Autodesk Inventor part; units mm, degrees
ref_plane "Work Plane1" through (33.5, 0, 0) normal (1, 0, 0) x (0, 1, 0)
ref_plane "XZ Plane" through (0, 0, 0) normal (0, 1, 0) x (-1, 0, 0)
ref_plane "XY Plane" through (0, 0, 0) normal (0, 0, 1) x (1, 0, 0)
sketch "Sketch1" plane through (0, 0, 0) normal (0, 1, 0) x (-1, 0, 0)
  circle A0 centre (0, 0) radius 33.5
  dimension "d0" = 67
extrude "Extrusion1" add sketch "Sketch1" along normal blind 6
ref_plane "Work Plane1" through (33.5, 0, 0) normal (1, 0, 0) x (0, 1, 0)
sketch "Sketch6" plane through (33.5, 0, 0) normal (1, 0, 0) x (0, 1, 0)
  line L0 (0, -33.5) -> (0, 33.5)
  point P0 (0, 0)
  point P1 (2.5, 0)
  dimension "d47" = 2.5
hole "Hole4" at (33.5, 2.5, 0) direction (-1, 0, 0) diameter 3 depth 8 tip angle 118
pattern_circular "Circular Pattern3" count 3 over 360 about axis through (0, 0, 0) along (0, 1, 0) of "Hole4"
sketch "Sketch7" plane through (0, 0, 0) normal (0, -1, 0) x (1, 0, 0)
  circle A0 centre (0, 0) radius 24.25
  circle A1 centre (0, 0) radius 33.5
  dimension "d58" = 48.5
  dimension "d59" = 67
extrude "Extrusion3" add sketch "Sketch7" along normal blind 3
chamfer "Chamfer1" distance 1.5 angle 45 1 edges at (-24.25, -3, 0)
sketch "Sketch8" plane through (0, 6, 0) normal (0, 1, 0) x (1, 0, 0)
  circle A0 centre (13.25, -22.9497) radius 1.5
  circle A1 centre (0, 0) radius 33.5 construction
  line L0 (0, 0) -> (13.25, -22.9497) construction
  line L1 (0, 0) -> (33.5, 0) construction
  dimension "d65" = 3
  dimension "d66" = 26.5
  dimension "d67" = 60
extrude "Extrusion4" cut sketch "Sketch8" against normal blind 10
pattern_circular "Circular Pattern4" count 3 over 360 about axis through (0, 0, 0) along (0, 1, 0) of "Extrusion4"
properties part number "Engine bulkhead" material "Steel AISI 1006 85 HR"
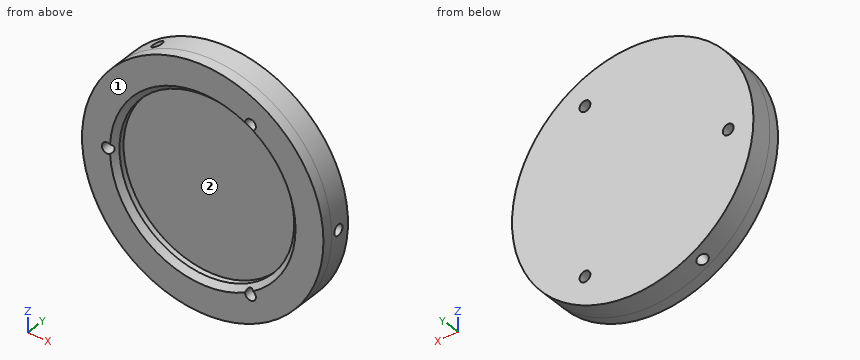
For this review, take the finished solid that the model builds, in its own axes (mm). Face numbers are marked on the shaded views. Round coordinates to 2 decimals unless told otherwise and drop trailing zeros. Loops run counter-clockwise (first coordinate to the right, second up) from the corner with the lowest first, then second, coordinate; pieces in that order, holes last. Notation, with made-up numbers: (-26.5, 55) - (4.5, 55) arc R31 ccw to (4.5, 79) - close; hole circle Ø1 at (88, 39.5). An arc over 180 degrees is marked (long way). Answer as CSV lines item,"result".
(1) Wall thickness on line 1 (Z direction, x = 13.25, y = 4.25); line 2 (X direction, y = 2.75, z = -23); line 3 (Z direction, x = 0, y = -1.1): over which ranges is each line inside the solid? List them lowest first.
Checked values:
line 1,"z = -30.77 to -24.45, -21.45 to 21.45, 24.45 to 30.77"
line 2,"x = -24.36 to -14.99, -11.57 to 11.75, 14.75 to 24.36"
line 3,"z = -33.5 to -24.25, 24.25 to 33.5"
(2) Mouldability with a two-part tool opening along X and no side actions: class the marked faces 1 and 2 as +X half, -X half, draft (parallel to the pull), parting line (faces both ways), or undercut.
Checked values:
face 1,"draft"
face 2,"undercut"
(3) Insertion check: P1, Ø1.5, axis at x = 13, y = 5, coming from the +Z side; P2, Ø5, axis at y = 1.5, z = 21, coming from the +X side; P3, Ø14.5, axis at x = 10, z = 1, coming from the -Y side. Each pin has a flat end and moves straight along its axis. Give the tip position at first contact, or say it passes through.
Checked values:
P1,"stops at z = 31.18"
P2,"stops at x = 27.93"
P3,"stops at y = 0"
(4) Consider section A-A on x = 0. Give the boundary of the cut face in (y, z), then the cut area to 3 significant figures.
Checked values:
outline,"(-3, -33.5) - (6, -33.5) - (6, 33.5) - (-3, 33.5) - (-3, 25.75) - (-1.5, 24.25) - (0, 24.25) - (0, -24.25) - (-1.5, -24.25) - (-3, -25.75) - close"
area,"455 mm2"
